Read the model definition and answer for the solid it produces. Units are mm, in the model's axes. Face numbers are marked on the shaded views. A direction names the side the tool comes from. Coordinates: 2 decimals unless noted, no trailing zeros. Write each loop counter-clockwise with the first axis right and the second up, starting at its lowest first coordinate (ties: lowest second). Pieces come first, ordered by that corner, then holes. Notation, with made-up numbers: M 83.25,81.5 L 137.25,81.5 A14 cw 137.25,95.5 Z; hole C -40,38.25 d9. An arc over 180 degrees is marked long. Write item = value, one per line.
Autodesk Inventor part; units mm, degrees
ref_plane "YZ Plane" through (0, 0, 0) normal (1, 0, 0) x (0, 1, 0)
ref_plane "XZ Plane" through (0, 0, 0) normal (0, 1, 0) x (-1, 0, 0)
ref_plane "XY Plane" through (0, 0, 0) normal (0, 0, 1) x (1, 0, 0)
sketch "Sketch1" plane through (0, 0, 0) normal (0, 1, 0) x (-1, 0, 0)
  line L0 (-39.6659, 82.3437) -> (-60.406, 61.6036)
  line L1 (-60.406, 61.6036) -> (-60.406, 8.9397)
  circle A0 centre (-37.593, 50.6893) radius 1.75
  circle A1 centre (-37.593, 50.6893) radius 1.75
  line L2 (-60.406, 8.9397) -> (-40.093, 8.9397)
  line L3 (-40.093, 47) -> (-33.9037, 47)
  line L4 (-33.9037, 47) -> (-33.9037, 59.379)
  line L5 (-25.3025, 67.9802) -> (-33.9037, 59.379)
  line L6 (-40.093, 47) -> (-40.093, 8.9397)
  line L7 (-39.6659, 82.3437) -> (-25.3025, 67.9802)
extrude "Extrusion1" add sketch "Sketch1" along normal blind 2
sketch "Sketch2" plane through (0, 2, 0) normal (0, 1, 0) x (1, 0, 0)
  line L0 (39.6659, -82.3437) -> (60.406, -61.6036)
  line L1 (60.406, -61.6036) -> (60.406, -8.9397)
  line L2 (60.406, -61.6036) -> (60.406, -46.6036)
  line L3 (60.406, -46.6036) -> (58.406, -46.6036)
  line L4 (58.406, -46.6036) -> (58.406, -60.7752)
  line L5 (60.406, -61.6036) -> (49.7994, -72.2102)
  line L6 (49.7994, -72.2102) -> (48.3852, -70.796)
  line L7 (48.3852, -70.796) -> (58.406, -60.7752)
  line L8 (60.406, -8.9397) -> (58.406, -8.9397)
  line L9 (58.406, -8.9397) -> (58.406, -23.9397)
  line L10 (58.406, -23.9397) -> (60.406, -23.9397)
  line L11 (60.406, -23.9397) -> (60.406, -8.9397)
  line L12 (39.6659, -82.3437) -> (44.9692, -77.0404)
  line L13 (44.9692, -77.0404) -> (43.555, -75.6262)
  line L14 (43.555, -75.6262) -> (38.2517, -80.9295)
  line L15 (38.2517, -80.9295) -> (39.6659, -82.3437)
  line L16 (39.6659, -82.3437) -> (47.1659, -82.3437) construction
  point P0 (0, 0)
  dimension "d6" = 15
  dimension "d7" = 2
  dimension "d8" = 15
  dimension "d9" = 2
  dimension "d10" = 90
  dimension "d11" = 90
  dimension "d12" = 15
  dimension "d13" = 7.5
  dimension "d14" = 45
  dimension "d15" = 2
extrude "Extrusion2" add sketch "Sketch2" along normal blind 15
properties part number "covfronti2c1"
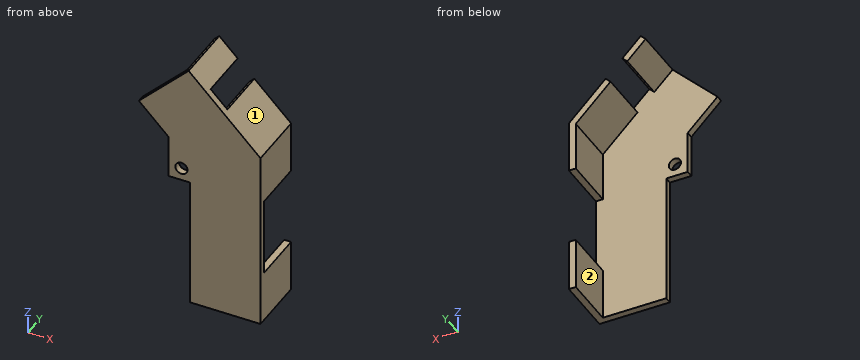
Item 1: Flat-ended cylindrical pins translate along their axes: pin 1 (1 mm diameter, centred on x = 40.5, z = 48.5, fed in from -Y); pin 2 (7.5 mm diameter, centred on y = 10, z = 14, fed in from -X); pin 3 (5.5 mm diameter, centred on x = 37.59, z = 50.69, fed in from +Y); pin 4 (2 mm diameter, centred on x = 59, y = 6.5, fed in from +Z). Find the tip coordinate at first contact, or state that the pin passes through.
Worked answers:
pin_1 = 0
pin_2 = 58.41
pin_3 = 2
pin_4 = 64.01
Item 2: Find section D-D (z = 22.5). Determine the outline of the cut face in (x, y), and give its area (3 significant figures).
Worked answers:
outline = M 40.09,0 L 60.41,0 L 60.41,17 L 58.41,17 L 58.41,2 L 40.09,2 Z
area = 70.6 mm²
Item 3: Consider line 1 along Y through (x, z) = (34.5, 48.5); line 2 along X through (y, z) = (6.5, 23.5); line 3 along Z through (x, y) = (59, 2.5). Determine where each line is inside the solid, lowest interval first. Write a range as from..to.
Worked answers:
line_1 = 0..2
line_2 = 58.41..60.41
line_3 = 8.94..23.94, 46.6..63.01
Item 4: Which of the six approach directions +Z, -Z, +X, -X, +Y, -Y give full straight-line access (tool end or side, diameter ignored) to the marked faces 1 and 2?
Worked answers:
face_1 = +Z, +X, +Y, -Y
face_2 = -Z, -X, +Y
Item 5: Find section C-C (x = 51.5). Determine the outline of the cut face in (y, z), and give its area (3 significant figures).
Worked answers:
outline = M 0,8.94 L 2,8.94 L 2,67.68 L 17,67.68 L 17,70.51 L 0,70.51 Z
area = 166 mm²
Item 6: Find section A-A (y = 8.75). Determine the outline of the cut face in (x, z) (1 decimal), and give its area (3 significant figures).
Worked answers:
outline = M 38.3,80.9 L 43.6,75.6 L 45,77 L 39.7,82.3 Z; M 48.4,70.8 L 58.4,60.8 L 58.4,46.6 L 60.4,46.6 L 60.4,61.6 L 49.8,72.2 Z; M 58.4,8.9 L 60.4,8.9 L 60.4,23.9 L 58.4,23.9 Z
area = 103 mm²
Item 7: Find section B-B (z = 34.5). Determine the outline of the cut face in (x, y), and give its area (3 significant figures).
Worked answers:
outline = M 40.09,0 L 60.41,0 L 60.41,2 L 40.09,2 Z
area = 40.6 mm²
